from build123d import *

# Parameters (mm, degrees)
SKETCH1_R           = 2.5
SKETCH1_R_2         = 1.625
BOSS_EXTRUDE1_DEPTH = 4
BOSS_EXTRUDE2_START = -4
SKETCH1_2_R         = 2.5
SKETCH1_2_R_2       = 1.625
BOSS_EXTRUDE2_DEPTH = 4
SKETCH2_W           = 0.25
SKETCH2_H           = 1
CUT_EXTRUDE1_DEPTH  = 9.746427842


with BuildPart() as part:
    # Sketch1 → Boss-Extrude1 (new body)
    with BuildSketch(Plane.XY):
        Circle(SKETCH1_R)
        Circle(SKETCH1_R_2, mode=Mode.SUBTRACT)
    extrude(amount=BOSS_EXTRUDE1_DEPTH)

    # Sketch1_2 → Boss-Extrude2 (add)
    # profile 1 of 2: a face of its own
    with BuildSketch(Plane.XY.offset(BOSS_EXTRUDE2_START)):
        Circle(SKETCH1_2_R)
        Circle(SKETCH1_2_R_2, mode=Mode.SUBTRACT)
    # profile 2 of 2: a face of its own
    with BuildSketch(Plane.XY.offset(BOSS_EXTRUDE2_START)):
        Circle(SKETCH1_2_R_2)
    extrude(amount=BOSS_EXTRUDE2_DEPTH)

    # Sketch2 → Cut-Extrude1 (cut, through all)
    with BuildSketch(Plane.XY.offset(4)):
        Polygon((0.355928439, 2.275728443), (0.56384013, 3.253876044), (0.80837703, 3.201898121), (0.600465339, 2.22375052), align=None)
        with Locations((0, 2.8)):
            Rectangle(SKETCH2_W, SKETCH2_H)
        Polygon((0.821301097, 2.151996633), (1.22803774, 3.065542091), (1.456424104, 2.96385793), (1.049687461, 2.050312472), align=None)
        Polygon((1.250778956, 1.934212244), (1.838564208, 2.743229238), (2.040818457, 2.596282925), (1.453033205, 1.787265931), align=None)
        Polygon((1.625591773, 1.631893498), (2.368736598, 2.301024104), (2.53601925, 2.115237898), (1.792874424, 1.446107291), align=None)
        Polygon((1.929358429, 1.258253175), (2.795383832, 1.758253175), (2.920383832, 1.541746825), (2.054358429, 1.041746825), align=None)
        Polygon((2.148802863, 0.829621152), (3.099859379, 1.138638146), (3.177113628, 0.900874017), (2.226057112, 0.591857023), align=None)
        Polygon((2.274334301, 0.364730702), (3.268856197, 0.469259166), (3.294988313, 0.220628692), (2.300466417, 0.116100229), align=None)
        Polygon((2.300466417, -0.116100229), (3.294988313, -0.220628692), (3.268856197, -0.469259166), (2.274334301, -0.364730702), align=None)
        Polygon((2.226057112, -0.591857023), (3.177113628, -0.900874017), (3.099859379, -1.138638146), (2.148802863, -0.829621152), align=None)
        Polygon((2.054358429, -1.041746825), (2.920383832, -1.541746825), (2.795383832, -1.758253175), (1.929358429, -1.258253175), align=None)
        Polygon((1.792874424, -1.446107291), (2.53601925, -2.115237898), (2.368736598, -2.301024104), (1.625591773, -1.631893498), align=None)
        Polygon((1.453033205, -1.787265931), (2.040818457, -2.596282925), (1.838564208, -2.743229238), (1.250778956, -1.934212244), align=None)
        Polygon((1.049687461, -2.050312472), (1.456424104, -2.96385793), (1.22803774, -3.065542091), (0.821301097, -2.151996633), align=None)
        Polygon((0.600465339, -2.22375052), (0.80837703, -3.201898121), (0.56384013, -3.253876044), (0.355928439, -2.275728443), align=None)
        with Locations((0, -2.8)):
            Rectangle(SKETCH2_W, SKETCH2_H)
        Polygon((-0.355928439, -2.275728443), (-0.56384013, -3.253876044), (-0.80837703, -3.201898121), (-0.600465339, -2.22375052), align=None)
        Polygon((-0.821301097, -2.151996633), (-1.22803774, -3.065542091), (-1.456424104, -2.96385793), (-1.049687461, -2.050312472), align=None)
        Polygon((-1.250778956, -1.934212244), (-1.838564208, -2.743229238), (-2.040818457, -2.596282925), (-1.453033205, -1.787265931), align=None)
        Polygon((-1.625591773, -1.631893498), (-2.368736598, -2.301024104), (-2.53601925, -2.115237898), (-1.792874424, -1.446107291), align=None)
        Polygon((-1.929358429, -1.258253175), (-2.795383832, -1.758253175), (-2.920383832, -1.541746825), (-2.054358429, -1.041746825), align=None)
        Polygon((-2.148802863, -0.829621152), (-3.099859379, -1.138638146), (-3.177113628, -0.900874017), (-2.226057112, -0.591857023), align=None)
        Polygon((-2.274334301, -0.364730702), (-3.268856197, -0.469259166), (-3.294988313, -0.220628692), (-2.300466417, -0.116100229), align=None)
        Polygon((-2.300466417, 0.116100229), (-3.294988313, 0.220628692), (-3.268856197, 0.469259166), (-2.274334301, 0.364730702), align=None)
        Polygon((-2.226057112, 0.591857023), (-3.177113628, 0.900874017), (-3.099859379, 1.138638146), (-2.148802863, 0.829621152), align=None)
        Polygon((-2.054358429, 1.041746825), (-2.920383832, 1.541746825), (-2.795383832, 1.758253175), (-1.929358429, 1.258253175), align=None)
        Polygon((-1.792874424, 1.446107291), (-2.53601925, 2.115237898), (-2.368736598, 2.301024104), (-1.625591773, 1.631893498), align=None)
        Polygon((-1.453033205, 1.787265931), (-2.040818457, 2.596282925), (-1.838564208, 2.743229238), (-1.250778956, 1.934212244), align=None)
        Polygon((-1.049687461, 2.050312472), (-1.456424104, 2.96385793), (-1.22803774, 3.065542091), (-0.821301097, 2.151996633), align=None)
        Polygon((-0.600465339, 2.22375052), (-0.80837703, 3.201898121), (-0.56384013, 3.253876044), (-0.355928439, 2.275728443), align=None)
    extrude(amount=-CUT_EXTRUDE1_DEPTH, mode=Mode.SUBTRACT)


solid = part.part
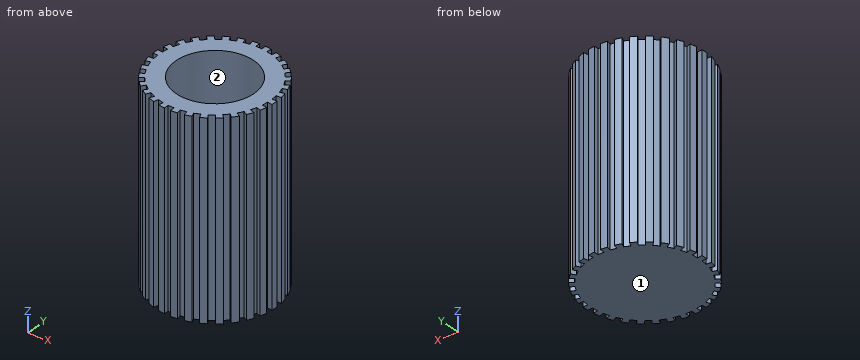
Geometry: final body of the model. Coordinates: model frame, mm. Face numbers are marked on the shaded views. Coordinates: 2 decimals unless noted, no trailing zeros. Loops run counter-clockwise (first coordinate to the right, second up) from the corner with the lowest first, then second, coordinate; pieces in that order, holes last. Notation, with made-up numbers: (50, -16) - (68, -16) arc R23 cw to (68, 3) - close; hole circle Ø8 at (31.5, 38). An arc over 180 degrees is marked (long way). Put each result on its own line as item: value. Start each with the question number.
Q1. Line query: line 1 (Y direction, x = 0, z = 1.7) (3 decimals); line 2 (Z direction, x = -0.1, y = -0.3); line 3 (X direction, y = 2, z = -0.75). Output: solid intervals per line, ascending.
Q2. Pin query (flat end, axial travel): pin 1 Ø1 at (y, z) = (-0.5, 2) entering from +X. Return the tip coordinate at first contact, or that it passes through.
Q3. Pull-direction query (Y, two-part tool) for the marked faces 1 and 2; classes: released by +Y, released by -Y, zero draft, split by the parting line, or undercut.
Q4. Cut plane A-A, the plane x = 0. Return loops of the section in (y, z) (3 decimals).
Q5. Cut plane B-B, the plane y = 0. Return loops of the section in (x, z) (3 decimals).
Filled sheet:
1. line 1: -2.3 to -1.625, 1.625 to 2.3
1. line 2: -4 to 0
1. line 3: -1.3 to 1.3
2. pin 1: x = 2.5
3. face 1: zero draft
3. face 2: undercut
4. outline: (-2.3, -4) - (2.3, -4) - (2.3, 4) - (1.625, 4) - (1.625, 0) - (-1.625, 0) - (-1.625, 4) - (-2.3, 4) - close
5. outline: (-2.5, -4) - (2.5, -4) - (2.5, 4) - (1.625, 4) - (1.625, 0) - (-1.625, 0) - (-1.625, 4) - (-2.5, 4) - close
